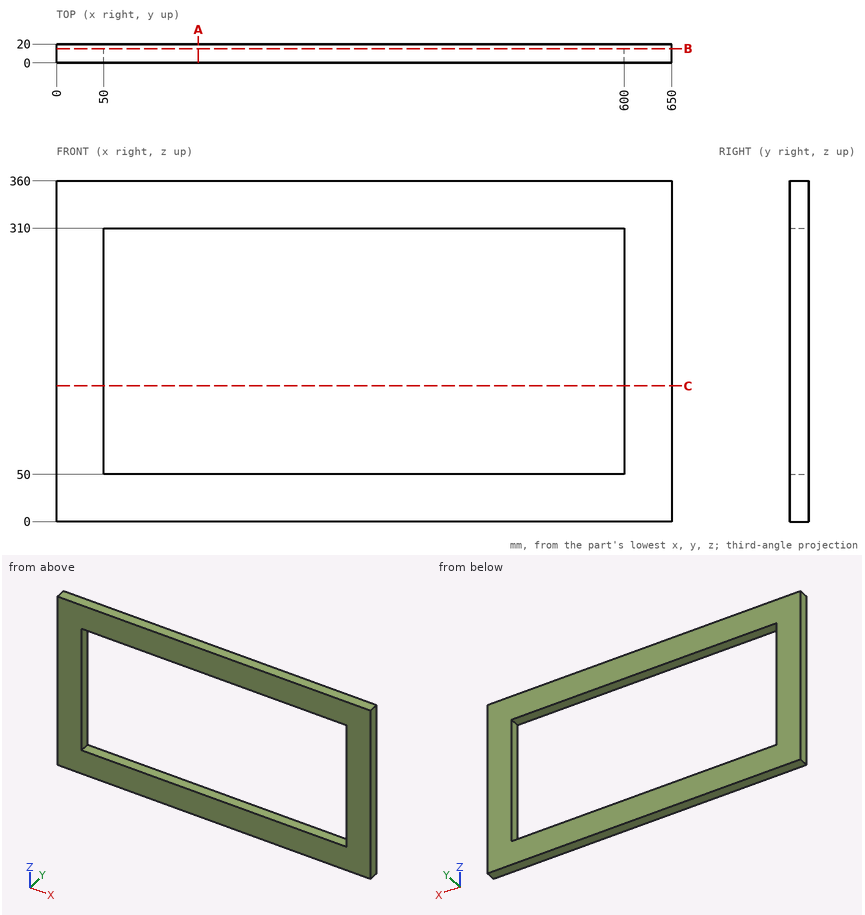
Source: three-view drawing plus pictorial views. Frame: mm from the lowest corner of the part. Give positions to 0.01 mm unless a question says otherwise; leave off trailing zeros. Order: outer loops, then holes, each group sorted by start corner. A loop starts at its lowest first (then second) coordinate and runs counter-clockwise, first axis right, second up. Notation, with made-up numbers: M -32,84.5 L 11,84.5 A26 cw 11,101.5 Z; hole C 43,31 d11. An arc over 180 degrees is marked long. One line per question, with ' | ' between items. Start each with the question number.
1. Section query A-A (x = 150). Return the cut outline in (y, z).
2. First-contact query: pin 1 Ø1 at (x, y) = (298.5, 10.5) entering from -Z. Flat tip, straight axial feed; report the tip coordinate or a pass-through.
3. Section query C-C (z = 143.5). Return the cut outline in (x, y).
4. Section query B-B (y = 15). Return the cut outline in (x, z).
5. Material intervals for probe 1 along Z at (x, y) = (387, 17); probe 2 along X at (y, z) = (4, 185), sorted ascending. Write a range as [from, to].
Here are the results:
1) outline: M 0,0 L 20,0 L 20,50 L 0,50 Z; M 0,310 L 20,310 L 20,360 L 0,360 Z
2) pin 1: z = 0
3) outline: M 0,0 L 50,0 L 50,20 L 0,20 Z; M 600,0 L 650,0 L 650,20 L 600,20 Z
4) outline: M 0,0 L 650,0 L 650,360 L 0,360 Z; hole M 50,50 L 600,50 L 600,310 L 50,310 Z
5) probe 1: [0, 50], [310, 360] | probe 2: [0, 50], [600, 650]
